```python
from build123d import *

# Parameters (mm, degrees)
EXTRUDE_1_DEPTH          = 2
SKETCH_3_W               = 76.4
SKETCH_3_H               = 2
EXTRUDE_2_DEPTH          = 7
CUT_EXTRUDE_1_DEPTH      = 10
EXTRUDE_4_DEPTH          = 2
PATTERN_LINEAR_2_COUNT   = 2
PATTERN_LINEAR_2_PITCH   = 32
FILLET_3_R               = 0.5
CUT_EXTRUDE_2_DEPTH      = 10
EXTRUDE_5_DEPTH          = 2
CUT_EXTRUDE_3_DEPTH      = 10
CUT_EXTRUDE_4_DEPTH      = 10
FILLET_5_R               = 2
EXTRUDE_9_DEPTH          = 2
FILLET_6_R               = 2
FILLET_7_R               = 1
SKETCH_18_W              = 76.4
SKETCH_18_H              = 2
EXTRUDE_6_DEPTH          = 2
SKETCH_19_W              = 10
SKETCH_19_H              = 10
CUT_EXTRUDE_5_DEPTH      = 3
EXTRUDE_8_DEPTH          = 2
FILLET_8_R               = 2
FILLET_9_R               = 2
SKETCH_21_W              = 3
SKETCH_21_H              = 87.342834434
CUT_EXTRUDE_6_DEPTH      = 3
CUT_EXTRUDE_7_DEPTH      = 1
CUT_EXTRUDE_7_DEPTH_BACK = 3
SKETCH_24_W              = 15
SKETCH_24_H              = 2
EXTRUDE_10_DEPTH         = 3
SKETCH_25_R              = 1
CUT_EXTRUDE_8_DEPTH      = 3


with BuildPart() as part:
    # 草图1 → 凸台-拉伸1 (new body)
    with BuildSketch(Plane(origin=(0, 0, 0), x_dir=(1, 0, 0), z_dir=(0, 1, 0))):
        with BuildLine():
            Line((-38.2, -44.69), (-38.2, -45.85))
            Line((-38.2, -45.85), (38.2, -45.85))
            Line((38.2, -45.85), (38.2, 45.85))
            Line((38.2, 45.85), (-38.2, 45.85))
            Line((-38.2, 45.85), (-38.2, 39.31))
            ThreePointArc((-38.2, 39.31), (3.8, -2.69), (-38.2, -44.69))
        make_face()
    extrude(amount=EXTRUDE_1_DEPTH)

    # 草图3 → 凸台-拉伸2 (add)
    with BuildSketch(Plane(origin=(0, 0, -45.85), x_dir=(-1, 0, 0), z_dir=(0, 0, -1))):
        with Locations((0, 1)):
            Rectangle(SKETCH_3_W, SKETCH_3_H)
    extrude(amount=EXTRUDE_2_DEPTH)

    # 草图5 → 切除-拉伸1 (cut)
    with BuildSketch(Plane(origin=(0, 2, 0), x_dir=(1, 0, 0), z_dir=(0, 1, 0))):
        Polygon((-38.2, 51.26), (38.2, 52.85), (-38.2, 52.85), align=None)
    extrude(amount=-CUT_EXTRUDE_1_DEPTH, mode=Mode.SUBTRACT)

    # 草图7 → 凸台-拉伸4 (add)
    with BuildSketch(Plane.XZ):
        Polygon((25.6, -52.587774869), (25.6, -54.754790576), (9.6, -54.754790576), (9.6, -52.254790576), align=None)
    extrude_4 = extrude(amount=-EXTRUDE_4_DEPTH)

    # 阵列(线性)2: 凸台-拉伸4 ×2
    with Locations(*[Vector(-0.999783511, 0, 0.020807013) * (i * PATTERN_LINEAR_2_PITCH) for i in range(1, PATTERN_LINEAR_2_COUNT)]):
        add(extrude_4)

    # 圆角3
    fillet_3_edges = [part.edges().sort_by_distance(p)[0] for p in [
        (25.6, 1, -54.754790576),
        (9.6, 1, -54.754790576),
        (-6.393072342, 1, -54.088966165),
        (-22.393072342, 1, -54.088966165),
    ]]
    fillet(fillet_3_edges, radius=FILLET_3_R)

    # 草图10 → 切除-拉伸2 (cut)
    with BuildSketch(Plane(origin=(0, 2, 0), x_dir=(1, 0, 0), z_dir=(0, 1, 0))):
        Polygon((-38.882265213, 53.905585721), (39.585789662, 55.538625083), (39.585789662, 48.538625083), (-38.2, 46.919784696), (-39.22769149, 52.889737929), align=None)
    extrude(amount=-CUT_EXTRUDE_2_DEPTH, mode=Mode.SUBTRACT)

    # 草图11 → 凸台-拉伸5 (add)
    with BuildSketch(Plane(origin=(0, 2, 0), x_dir=(1, 0, 0), z_dir=(0, 1, 0))):
        Polygon((-38.2, 46.919784696), (38.2, 49.509784696), (38.2, 48.509784696), align=None)
    extrude(amount=-EXTRUDE_5_DEPTH)

    # 草图13 → 切除-拉伸3 (cut)
    with BuildSketch(Plane.XZ):
        Polygon((38.2, -49.509784696), (37.7, -49.492834434), (38.2, 45.85), align=None)
    extrude(amount=-CUT_EXTRUDE_3_DEPTH, mode=Mode.SUBTRACT)

    # 草图16 → 切除-拉伸4 (cut)
    with BuildSketch(Plane.XZ):
        with BuildLine():
            ThreePointArc((-21.63159016, -39.14883119), (-26.948214114, -40.880601492), (-32.438562967, -41.939652064))
            Line((-32.438562967, -41.939652064), (32.727956442, -44.14883119))
            Line((32.727956442, -44.14883119), (32.754177605, -39.14883119))
            Line((32.754177605, -39.14883119), (-21.63159016, -39.14883119))
        make_face()
        with BuildLine():
            ThreePointArc((-6.399232266, -29.14883119), (-9.26951053, -31.777764346), (-12.35622867, -34.14883119))
            Line((-12.35622867, -34.14883119), (32.780398767, -34.14883119))
            Line((32.780398767, -34.14883119), (32.80661993, -29.14883119))
            Line((32.80661993, -29.14883119), (-6.399232266, -29.14883119))
        make_face()
        with BuildLine():
            ThreePointArc((1.145462918, -19.14883119), (-0.38438284, -21.702193399), (-2.079685213, -24.14883119))
            Line((-2.079685213, -24.14883119), (32.832841093, -24.14883119))
            Line((32.832841093, -24.14883119), (32.859062256, -19.14883119))
            Line((32.859062256, -19.14883119), (1.145462918, -19.14883119))
        make_face()
        with BuildLine():
            ThreePointArc((5.214767949, -9.14883119), (4.446089194, -11.673532869), (3.530729255, -14.14883119))
            Line((3.530729255, -14.14883119), (32.885283419, -14.14883119))
            Line((32.885283419, -14.14883119), (32.911504582, -9.14883119))
            Line((32.911504582, -9.14883119), (5.214767949, -9.14883119))
        make_face()
        with BuildLine():
            Line((32.937725745, -4.14883119), (32.963946908, 0.85116881))
            Line((32.963946908, 0.85116881), (6.762414302, 0.85116881))
            ThreePointArc((6.762414302, 0.85116881), (6.58968308, -1.65560578), (6.277301941, -4.14883119))
            Line((6.277301941, -4.14883119), (32.937725745, -4.14883119))
        make_face()
        with BuildLine():
            Line((33.016389234, 10.85116881), (6.053760559, 10.85116881))
            ThreePointArc((6.053760559, 10.85116881), (6.441352349, 8.360067057), (6.688829476, 5.85116881))
            Line((6.688829476, 5.85116881), (32.990168071, 5.85116881))
            Line((32.990168071, 5.85116881), (33.016389234, 10.85116881))
        make_face()
        with BuildLine():
            Line((33.06883156, 20.85116881), (2.97246589, 20.85116881))
            ThreePointArc((2.97246589, 20.85116881), (3.976569254, 18.378754125), (4.832355682, 15.85116881))
            Line((4.832355682, 15.85116881), (33.042610397, 15.85116881))
            Line((33.042610397, 15.85116881), (33.06883156, 20.85116881))
        make_face()
        with BuildLine():
            Line((33.121273886, 30.85116881), (-3.100875064, 30.85116881))
            ThreePointArc((-3.100875064, 30.85116881), (-1.274777634, 28.410185715), (0.381864384, 25.85116881))
            Line((0.381864384, 25.85116881), (33.095052723, 25.85116881))
            Line((33.095052723, 25.85116881), (33.121273886, 30.85116881))
        make_face()
        with BuildLine():
            Line((33.173710083, 40.85), (-14.350169812, 40.85))
            ThreePointArc((-14.350169812, 40.85), (-10.950539992, 38.501547429), (-7.780649528, 35.85116881))
            Line((-7.780649528, 35.85116881), (33.147495049, 35.85116881))
            Line((33.147495049, 35.85116881), (33.173710083, 40.85))
        make_face()
    extrude(amount=-CUT_EXTRUDE_4_DEPTH, mode=Mode.SUBTRACT)

    # 圆角5
    fillet_5_edges = [part.edges().sort_by_distance(p)[0] for p in [
        (-21.63159016, 1, -39.14883119),
        (32.754177605, 1, -39.14883119),
        (32.727956442, 1, -44.14883119),
        (-6.399232266, 1, -29.14883119),
        (32.80661993, 1, -29.14883119),
        (32.780398767, 1, -34.14883119),
        (-2.079685213, 1, -24.14883119),
        (3.530729255, 1, -14.14883119),
        (5.214767949, 1, -9.14883119),
        (32.911504582, 1, -9.14883119),
        (32.885283419, 1, -14.14883119),
        (32.937725745, 1, -4.14883119),
        (6.688829476, 1, 5.85116881),
        (33.016389234, 1, 10.85116881),
        (32.990168071, 1, 5.85116881),
        (4.832355682, 1, 15.85116881),
        (2.97246589, 1, 20.85116881),
        (0.381864384, 1, 25.85116881),
        (-3.100875064, 1, 30.85116881),
        (33.121273886, 1, 30.85116881),
        (-14.350169812, 1, 40.85),
        (33.173710083, 1, 40.85),
    ]]
    fillet(fillet_5_edges, radius=FILLET_5_R)

    # 草图23 → 凸台-拉伸9 (add)
    with BuildSketch(Plane.XZ):
        with BuildLine():
            Line((30.743661638, -39.14883119), (-21.254296123, -39.14883119))
            ThreePointArc((-21.254296123, -39.14883119), (-21.621062836, -39.182748237), (-21.975389905, -39.283349012))
            ThreePointArc((-21.975389905, -39.283349012), (-27.127035015, -40.926389654), (-32.438562967, -41.939652064))
            Line((-32.438562967, -41.939652064), (30.67101495, -44.079099797))
            ThreePointArc((30.67101495, -44.079099797), (32.125051399, -43.521859473), (32.738749569, -42.090736373))
            Line((32.738749569, -42.090736373), (32.743634136, -41.159319511))
            ThreePointArc((32.743634136, -41.159319511), (32.161578532, -39.738330684), (30.743661638, -39.14883119))
        make_face()
    extrude(amount=-EXTRUDE_9_DEPTH)

    # 圆角6
    fillet_6_edges = [part.edges().sort_by_distance(p)[0] for p in [
        (-12.35622867, 1, -34.14883119),
        (1.145462918, 1, -19.14883119),
        (32.859062256, 1, -19.14883119),
        (32.832841093, 1, -24.14883119),
        (6.277301941, 1, -4.14883119),
        (6.762414302, 1, 0.85116881),
        (32.963946908, 1, 0.85116881),
        (6.053760559, 1, 10.85116881),
        (33.06883156, 1, 20.85116881),
        (33.042610397, 1, 15.85116881),
        (33.095052723, 1, 25.85116881),
        (-7.780649528, 1, 35.85116881),
        (33.147495049, 1, 35.85116881),
    ]]
    fillet(fillet_6_edges, radius=FILLET_6_R)

    # 圆角7
    fillet_7_edges = [part.edges().sort_by_distance(p)[0] for p in [
        (-38.2, 1, 44.69),
        (-38.2, 1, -39.31),
        (-38.2, 1, -46.919784696),
    ]]
    fillet(fillet_7_edges, radius=FILLET_7_R)

    # 草图18 → 凸台-拉伸6 (add)
    with BuildSketch(Plane.XY.offset(45.85)):
        with Locations((0, 1)):
            Rectangle(SKETCH_18_W, SKETCH_18_H)
    extrude(amount=EXTRUDE_6_DEPTH)

    # 草图19 → 切除-拉伸5 (cut, through all)
    with BuildSketch(Plane(origin=(0, 2, 0), x_dir=(1, 0, 0), z_dir=(0, 1, 0))):
        with Locations((33.2, -42.85)):
            Rectangle(SKETCH_19_W, SKETCH_19_H)
    extrude(amount=-CUT_EXTRUDE_5_DEPTH, mode=Mode.SUBTRACT)

    # 草图20 → 凸台-拉伸8 (add)
    with BuildSketch(Plane(origin=(0, 2, 0), x_dir=(1, 0, 0), z_dir=(0, 1, 0))):
        Polygon((25.2, -35.85116881), (33.157977385, -35.85116881), (33.157977385, -37.85), (28.2, -40.85), (25.2, -40.85), align=None)
    extrude(amount=-EXTRUDE_8_DEPTH)

    # 圆角8
    fillet_8_edges = [part.edges().sort_by_distance(p)[0] for p in [
        (25.2, 1, 40.85),
        (25.2, 1, 35.85116881),
    ]]
    fillet(fillet_8_edges, radius=FILLET_8_R)

    # 圆角9
    fillet_9_edges = [part.edges().sort_by_distance(p)[0] for p in [
        (33.157977385, 1, 37.85),
        (28.2, 1, 40.85),
    ]]
    fillet(fillet_9_edges, radius=FILLET_9_R)

    # 草图21 → 切除-拉伸6 (cut, through all)
    with BuildSketch(Plane.XZ):
        with Locations((36.658046139, -5.821417217)):
            Rectangle(SKETCH_21_W, SKETCH_21_H)
    extrude(amount=-CUT_EXTRUDE_6_DEPTH, mode=Mode.SUBTRACT)

    # 草图22 → 切除-拉伸7 (cut, two sides)
    with BuildSketch(Plane.XZ) as cut_extrude_7_sk:
        Polygon((-290.579437235, -45.15), (-39.244125604, -45.15), (60.755874396, -45.15), (60.755874396, -51.15), (-39.244125604, -51.15), (-39.244125604, -47.15), (-39.244125604, 204.185311631), (314.77499341, -152.673510404), (63.439681778, -402.008822036), align=None)
    extrude(amount=CUT_EXTRUDE_7_DEPTH, mode=Mode.SUBTRACT)
    extrude(cut_extrude_7_sk.sketch, amount=-CUT_EXTRUDE_7_DEPTH_BACK, mode=Mode.SUBTRACT)

    # 草图24 → 凸台-拉伸10 (add)
    with BuildSketch(Plane(origin=(0, 0, -45.15), x_dir=(-1, 0, 0), z_dir=(0, 0, -1))):
        with Locations((0, 1)):
            Rectangle(SKETCH_24_W, SKETCH_24_H)
    extrude_10 = extrude(amount=EXTRUDE_10_DEPTH)

    # 草图25 → 切除-拉伸8 (cut, through all)
    with BuildSketch(Plane(origin=(0, 2, 0), x_dir=(1, 0, 0), z_dir=(0, 1, 0))):
        with Locations((-8.5, 45.15)):
            Circle(SKETCH_25_R)
        with Locations((8.5, 45.15)):
            Circle(SKETCH_25_R)
    cut_extrude_8 = extrude(amount=-CUT_EXTRUDE_8_DEPTH, mode=Mode.SUBTRACT)

    # 镜向1: 凸台-拉伸10, 切除-拉伸8 across plane
    add(extrude_10.mirror(Plane.XY.offset(1.35)))
    add(cut_extrude_8.mirror(Plane.XY.offset(1.35)), mode=Mode.SUBTRACT)


solid = part.part
```
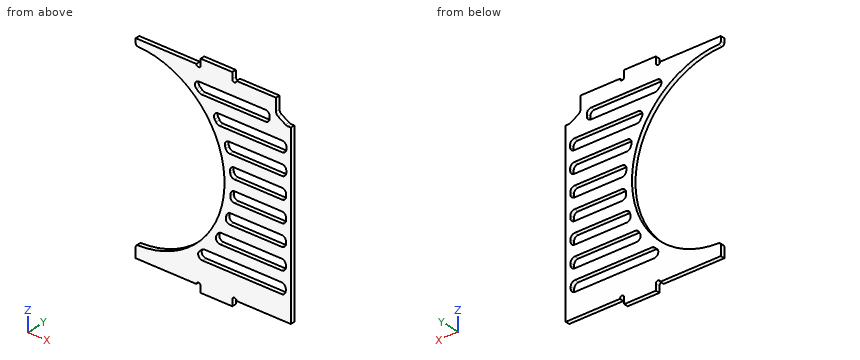
Can you work these out from the model? Positions are in its coordinate system, mm. Give positions to 0.01 mm unless a question says otherwise; leave off trailing zeros. Loops run counter-clockwise (first coordinate to the right, second up) from the corner with the lowest first, then second, coordinate; pieces in that order, holes last. Notation, with made-up numbers: M 26.25,-20 L 75.25,-20 A4 cw 75.25,-16 Z; hole C 86.25,0 d7. An arc over 180 degrees is marked long. Use CSV: the item, a comma, the result in double quotes. Start each with the question number.
1. Imagine slicing it at B-B, the plane z = 2.69. Write out the boundary of the cut face in (x, y).
2. Imagine slicing it at C-C, the plane x = 21.5. Count the separate pieces of the cut face and the enclosed holes in it, plus the area to 3 significant figures.
3. If I drill on L1, parallel to Z at x = -5, y = 1.5; L2, parallel to Z at x = -3, y = 0.55; L3, parallel to Z at x = -9, y = 1.2, over which ranges is the centre line in solid material (lowest first)?
4. Imagine slicing it at A-A, the plane x = -23.5. Write out the boundary of the cut face in (y, z).
5. For P1, Ø1, axis at x = -22, y = 0.5, coming from the -Z side; P2, Ø0.6, axis at x = 23, y = 1, coming from the +Z side; P3, Ø1, axis at y = 1.5, z = 49, coming from the +X side, each with a flat end and sliding along its axis, tell me the tip position at first contact or that it passes through.
Response values:
1,outline,"M 3.8,0 L 35.16,0 L 35.16,2 L 3.8,2 Z"
2,separate pieces,"9"
2,enclosed holes,"0"
2,area,"106 mm^2"
3,L1,"-48.15 to -34.15, -29.15 to -23.03, 28.41 to 35.85, 40.85 to 50.85"
3,L2,"-48.15 to -34.15, -29.15 to -20.22, 25.6 to 35.85, 40.85 to 50.85"
3,L3,"-44.28 to -27.5, 32.88 to 36.93, 40.67 to 46.98"
4,outline,"M 0,-45.15 L 2,-45.15 L 2,-36.65 L 0,-36.65 Z; M 0,42.03 L 2,42.03 L 2,47.85 L 0,47.85 Z"
5,P1,"z = -45.15"
5,P2,"z = 47.85"
5,P3,"x = 7.5"
